from build123d import *

# Parameters (mm, degrees)
BOSS_EXTRUDE1_DEPTH = 22
SKETCH1_3_W         = 30
SKETCH1_3_H         = 10
BOSS_EXTRUDE2_DEPTH = 44
SKETCH1_4_W         = 30
SKETCH1_4_H         = 10
BOSS_EXTRUDE3_DEPTH = 52
SKETCH1_5_W         = 20
SKETCH1_5_H         = 10
BOSS_EXTRUDE4_DEPTH = 52


with BuildPart() as part:
    # Sketch1 → Boss-Extrude1 (new body)
    with BuildSketch(Plane.XY):
        Polygon((90, 0), (0, 0), (0, -110), (30, -110), (30, -120), (120, -120), (140, -100), (140, -10), (110, -10), (90, -10), align=None)
    extrude(amount=BOSS_EXTRUDE1_DEPTH)

    # Sketch1<3> → Boss-Extrude2 (add)
    with BuildSketch(Plane.XY):
        with Locations((15, -115)):
            Rectangle(SKETCH1_3_W, SKETCH1_3_H)
    extrude(amount=BOSS_EXTRUDE2_DEPTH)

    # Sketch1<4> → Boss-Extrude3 (add)
    with BuildSketch(Plane.XY):
        with Locations((125, -5)):
            Rectangle(SKETCH1_4_W, SKETCH1_4_H)
    extrude(amount=BOSS_EXTRUDE3_DEPTH)

    # Sketch1<5> → Boss-Extrude4 (add)
    with BuildSketch(Plane.XY):
        with Locations((100, -5)):
            Rectangle(SKETCH1_5_W, SKETCH1_5_H)
    extrude(amount=BOSS_EXTRUDE4_DEPTH)


solid = part.part
Design review of the part built by this model. Coordinates are the model's own, in mm. A direction names the side the tool comes from. Coordinates: 2 decimals unless noted, no trailing zeros. Loops run counter-clockwise (first coordinate to the right, second up) from the corner with the lowest first, then second, coordinate; pieces in that order, holes last. Notation, with made-up numbers: M 89,83 L 138,83 A24 cw 138,113 Z; hole C -10.5,31.25 d10. An arc over 180 degrees is marked long. Answer as CSV lines item,"result".
Item 1: Add section D-D on y = -19. State the section outline as (x, z) points.
Answer list:
outline,"M 0,0 L 140,0 L 140,22 L 0,22 Z"
Item 2: Add section C-C on z = 47. State the section outline as (x, y) points.
Answer list:
outline,"M 90,-10 L 140,-10 L 140,0 L 90,0 Z"
Item 3: Add section A-A on z = 32.5. State the section outline as (x, y) points, plus the area to 3 significant figures.
Answer list:
outline,"M 0,-120 L 30,-120 L 30,-110 L 0,-110 Z; M 90,-10 L 140,-10 L 140,0 L 90,0 Z"
area,"800 mm²"
Item 4: Add section B-B on x = 19. State the section outline as (y, z) points.
Answer list:
outline,"M -120,0 L 0,0 L 0,22 L -110,22 L -110,44 L -120,44 Z"
Item 5: For P1, Ø11, axis at x = 14, y = -115, coming from the +Z side; P2, Ø11, axis at y = -5.5, z = 34.5, coming from the -X side; P3, Ø11, axis at x = 17.5, z = 29.5, coming from the +Y side, all flat-tipped, find the tip position at first contact; note any pin that passes through.
Answer list:
P1,"z = 44"
P2,"x = 90"
P3,"y = -110"
Item 6: Machinability: for faces 1 (the face through (15, -110, 33)), 2 (the face through (115, -10, 37)), 3 (the face through (30, -115, 33)), which of the approach directions +Z, -Z, +X, -X, +Y, -Y give a long, thin tool a straight path to every point of the face, cutting with its end or side? Answer none if there is none.
Answer list:
face 1,"+Z, +X, -X, +Y"
face 2,"+Z, +X, -X, -Y"
face 3,"+Z, +X, +Y, -Y"
Item 7: For probe 1 along Y at (x, z) = (106, 29); probe 2 along Z at (x, y) = (11, -108); probe 3 along Y at (x, z) = (28, 42.5), list the stretches that pass through material, from the lowest coordinate up.
Answer list:
probe 1,"-10 to 0"
probe 2,"0 to 22"
probe 3,"-120 to -110"
